Read the model definition and answer for the solid it produces. Units are mm, in the model's axes. A direction names the side the tool comes from. Round coordinates to 2 decimals unless told otherwise and drop trailing zeros. Write each loop counter-clockwise with the first axis right and the second up, starting at its lowest first coordinate (ties: lowest second). Pieces come first, ordered by that corner, then holes. Notation, with made-up numbers: (35, 15.5) - (75, 15.5) arc R25 cw to (75, 29.5) - close; hole circle Ø5 at (-28.75, 8). An arc over 180 degrees is marked (long way). Use one line per item in the form item = value. Start each with the question number.
1) Each of these flat-tipped pins is pushed along its axis until it touches: pin 1 (4 mm diameter, centred on x = 4.5, y = 82.5, fed in from -Z); pin 2 (4 mm diameter, centred on x = 7.5, z = -432.5, fed in from +Y); pin 3 (6 mm diameter, centred on x = 7.5, z = -503, fed in from +Y); pin 4 (10 mm diameter, centred on x = 8, y = 113, fed in from +Z). Where does it stop, or does it pass through?
2) For faces 1 (the face through (14.93, 13.639, -860.596)), 2 (the face through (6.2, 108.5, -296.1)), determine the directions among +Z, -Z, +X, -X, +Y, -Y from which every point of the face is accessible in a straight line to the end or side of a thin tool.
3) The part is cut by section C-C, the plane z = -814. Give the vertices of the cut face in (x, y).
4) For a pull along Z with two mould halves and no side action, classify faces 3 (the face through (6.2, 108.5, -16.1)), 4 (the face through (6.2, 108.5, -436.1)), 5 (the face through (15, 27.666, -426)) as released by +Z, released by -Z, zero draft, split by the parting line, or undercut.
5) The part is cut by section A-A, the plane x = 13.5. Give the vertices of the cut face in (y, z).
6) Consider line 1 along X through (y, z) = (29.5, -555.5); line 2 along Y through (x, z) = (10.75, -749); line 3 along Z through (x, y) = (14.75, 17.5). Determine where each line is inside the solid, lowest interval first. Write a range as from..to.
from build123d import *

# Parameters (mm, degrees)
BOSS_EXTRUDE1_DEPTH = 10
BOSS_EXTRUDE2_DEPTH = 164
LPATTERN1_COUNT     = 10
LPATTERN1_PITCH     = 70


with BuildPart() as part:
    # Sketch5 → Boss-Extrude1 (new body)
    with BuildSketch(Plane(origin=(10, 0, 0), x_dir=(0, 0, -1), z_dir=(1, 0, 0))):
        Polygon((1000, 220), (1000, 0), (881.128856778, 0), (839.480242444, 27.665735559), (0, 27.665735559), (0, 192.334264441), (839.480242444, 192.334264441), (881.128856778, 220), align=None)
    extrude(amount=BOSS_EXTRUDE1_DEPTH)

    # Sketch6 → Boss-Extrude2 (add)
    with BuildSketch(Plane(origin=(0, 27.665735559, 0), x_dir=(-1, 0, 0), z_dir=(0, -1, 0))):
        Polygon((-10, 23.738513139), (-2.5, 23.738513139), (-10, 8.259066754), align=None)
    boss_extrude2 = extrude(amount=-BOSS_EXTRUDE2_DEPTH)

    # LPattern1: Boss-Extrude2 ×10
    with Locations(*[(0, 0, -i * LPATTERN1_PITCH) for i in range(1, LPATTERN1_COUNT)]):
        add(boss_extrude2)


solid = part.part
Geometry results:
q1.pin_1 = -653.74
q1.pin_2 = 191.67
q1.pin_3 = 192.33
q1.pin_4 = 0
q2.face_1 = +Z, +X, -X, -Y
q2.face_2 = -X, +Y, -Y
q3.outline = (10, 27.67) - (20, 27.67) - (20, 192.33) - (10, 192.33) - close
q4.face_3 = released by +Z
q4.face_4 = undercut
q4.face_5 = zero draft
q5.outline = (0, -1000) - (220, -1000) - (220, -881.13) - (192.33, -839.48) - (192.33, 0) - (27.67, 0) - (27.67, -839.48) - (0, -881.13) - close
q6.line_1 = 10..20
q6.line_2 = 27.67..192.33
q6.line_3 = -1000..-854.78
